```python
from build123d import *

# Parameters (mm, degrees)
F1_DEPTH = 952.5
F2_R     = 4
F3_DEPTH = 120.001


with BuildPart() as f1:
    # F0 (on Right) → F1 (new body)
    with BuildSketch(Plane.YZ):
        Polygon((-60, 13), (-60, 0), (60, 0), (60, 13), (6.5, 13), (6.5, 120), (-6.5, 120), (-6.5, 13), align=None)
    extrude(amount=-F1_DEPTH)

    # F2 (on Top) → F3 (cut, through all)
    with BuildSketch(Plane.XY):
        with Locations((-200, -46.0375)):
            Circle(F2_R)
        with Locations((-200, 46.0375)):
            Circle(F2_R)
        with Locations((-266.675, 46.0375)):
            Circle(F2_R)
        with Locations((-266.675, -46.0375)):
            Circle(F2_R)
        with Locations((-752.5, -46.0375)):
            Circle(F2_R)
        with Locations((-685.825, -46.0375)):
            Circle(F2_R)
        with Locations((-685.825, 46.0375)):
            Circle(F2_R)
        with Locations((-752.5, 46.0375)):
            Circle(F2_R)
    extrude(amount=F3_DEPTH, mode=Mode.SUBTRACT)


solid = f1.part
```
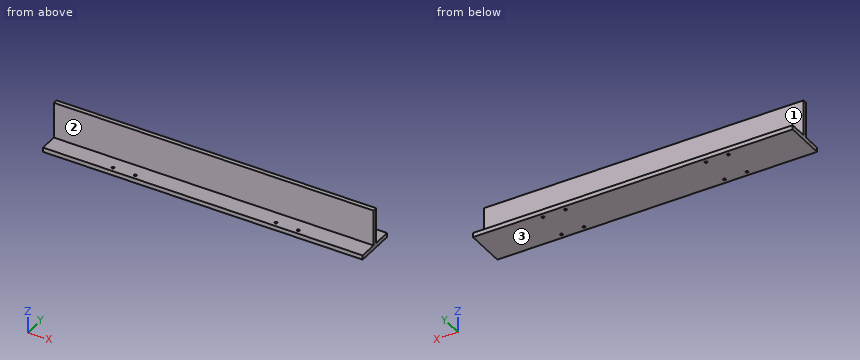
Input: part model. Units: mm. Frame: model coordinates. Face numbers are marked on the shaded views. A direction names the side the tool comes from. Give positions to 0.01 mm unless a question says otherwise; leave off trailing zeros. Loops run counter-clockwise (first coordinate to the right, second up) from the corner with the lowest first, then second, coordinate; pieces in that order, holes last.
1) Section query C-C on y = -14.5. Return the cut outline in (x, z), and give its area (3 significant figures).
A:
outline: (-952.5, 0) - (0, 0) - (0, 13) - (-952.5, 13) - close
area: 12,400 mm2
2) Line query: L1, parallel to Y at x = -752.5, z = 6; L2, parallel to X at y = 44.5, z = 10; L3, parallel to Y at x = -463, z = 88. Output: solid intervals per line, ascending.
A:
L1: y = -60 to -50.04, -42.04 to 42.04, 50.04 to 60
L2: x = -952.5 to -756.19, -748.81 to -689.52, -682.13 to -270.37, -262.98 to -203.69, -196.31 to 0
L3: y = -6.5 to 6.5
3) Contact query for flat-ended pins moving along their axis: pin 1 (9 mm diameter, centred on x = -200, y = -46.04, fed in from -Z); pin 2 (13 mm diameter, centred on x = -685.82, y = -46.04, fed in from +Z). Output: stop coordinate, or through.
A:
pin 1: stops at z = 0
pin 2: stops at z = 13
4) Reachability of the marked faces 1, 2 and 3 from +Z, -Z, +X, -X, +Y, -Y: full face, straight path, thin tool, end or side. Return the list, or none.
A:
face 1: +Z, +X, -X, +Y
face 2: +Z, +X, -X, -Y
face 3: -Z, +X, -X, +Y, -Y
5) Section query B-B on z = 100. Return the cut outline in (x, y).
A:
outline: (-952.5, -6.5) - (0, -6.5) - (0, 6.5) - (-952.5, 6.5) - close
6) Section query A-A on x = -552. Return the cut outline in (y, z), and give its area (3 significant figures).
A:
outline: (-60, 0) - (60, 0) - (60, 13) - (6.5, 13) - (6.5, 120) - (-6.5, 120) - (-6.5, 13) - (-60, 13) - close
area: 2,950 mm2
